from build123d import *

# Parameters (mm, degrees)
PAD007_DEPTH         = 6.9
POCKET005_DEPTH      = 2.951
POCKET005_DEPTH_BACK = 2.951
CHAMFER008_SIZE      = 0.6


with BuildPart() as part:
    # Sketch018 → Pad007 (new body)
    with BuildSketch(Plane.XY):
        with BuildLine():
            ThreePointArc((2.2, -1.9653244007), (0, 2.95), (-2.2, -1.9653244007))
            Line((-2.2, -1.9653244007), (2.2, -1.9653244007))
        make_face()
    extrude(amount=PAD007_DEPTH)

    # Sketch019 → Pocket005 (cut, two sides)
    with BuildSketch(Plane.YZ) as pocket005_sk:
        Polygon((-1.9, 6.9), (-1.5, 5.9), (-1.5, 1.75), (-1.15, 1.4), (5, 1.4), (5, 6.9), align=None)
    extrude(amount=-POCKET005_DEPTH, mode=Mode.SUBTRACT)
    extrude(pocket005_sk.sketch, amount=POCKET005_DEPTH_BACK, mode=Mode.SUBTRACT)

    # Chamfer008
    chamfer008_edges = [part.edges().sort_by_distance(p)[0] for p in [
        (0, 2.95, 0),
        (0, -1.965324, 0),
    ]]
    chamfer(chamfer008_edges, length=CHAMFER008_SIZE)


with BuildPart() as part_1:
    # Body053 placement: moved
    add(part.part.moved(Location((0, 18, 0))))


solid = part_1.part
Read the model definition and answer for the solid it produces. Units are mm, in the model's axes. A direction names the side the tool comes from. Round coordinates to 2 decimals unless told otherwise and drop trailing zeros. Order: outer loops, then holes, each group sorted by start corner. A loop starts at its lowest first (then second) coordinate and runs counter-clockwise, first axis right, second up.
1) The part is cut by section A-A on x = 0. Write down the section's boundary in (y, z).
2) Straight lines are drawn through the part: L1, parallel to X at y = 17.9, z = 0.75; L2, parallel to Z at x = 2, y = 17.2; L3, parallel to Y at x = -0.35, z = 2.5. For each, find the intervals that lie inside material, in ascending order.
3) For faces 5 (the face through (0, 18, 1.4)), 6 (the face through (0.08, 20.51, 0.16)), determine the directions among +Z, -Z, +X, -X, +Y, -Y from which every point of the face is accessible in a straight line to the end or side of a thin tool.
4) The mould has two halves that part along Y. Classify faces 1 (the face through (0, 16.035, 4)), 2 (the face through (0, 19, 0)), 3 (the face through (2.34, 16.204, 2.102)), 4 (the face through (0, 16.5, 4)): released by +Y, released by -Y, zero draft, split by the parting line, or undercut.
5) The part is cut by section B-B on y = 18. Write down the section's boundary in (x, z).
6) The part is cut by section C-C on z = 4.5. Write down the section's boundary in (x, y), plus the area to 3 significant figures.
7) The part is cut by section D-D on z = 1. Write down the section's boundary in (x, y), plus the area to 3 significant figures.
8) Flat-ended cylindrical pins translate along their axes: pin 1 (1.2 mm diameter, centred on x = 0.5, y = 18, fed in from +Z); pin 2 (2 mm diameter, centred on y = 17, z = 4.5, fed in from +X); pin 3 (1 mm diameter, centred on x = -0.5, z = 5, fed in from +Y). Find the tip coordinate at first contact, or state that the pin passes through.
Resolved:
1. outline: (16.03, 0.6) - (16.63, 0) - (20.35, 0) - (20.95, 0.6) - (20.95, 1.4) - (16.85, 1.4) - (16.5, 1.75) - (16.5, 5.9) - (16.1, 6.9) - (16.03, 6.9) - close
2. L1: x = -2.95 to 2.95
2. L2: z = 0 to 1.4
2. L3: y = 16.03 to 16.5
3. face 5: +Z, +X, -X, +Y
3. face 6: -Z
4. face 1: released by -Y
4. face 2: zero draft
4. face 3: split by the parting line
4. face 4: released by +Y
5. outline: (-2.95, 0.6) - (-2.35, 0) - (2.35, 0) - (2.95, 0.6) - (2.95, 1.4) - (-2.95, 1.4) - close
6. outline: (-2.54, 16.5) arc R2.95 ccw to (-2.2, 16.03) - (2.2, 16.03) arc R2.95 ccw to (2.54, 16.5) - close
6. area: 2.22 mm2
7. outline: (-2.2, 16.03) - (2.2, 16.03) arc R2.95 ccw (long way) to start
7. area: 24.3 mm2
8. pin 1: stops at z = 1.4
8. pin 2: stops at x = 2.54
8. pin 3: stops at y = 16.5
